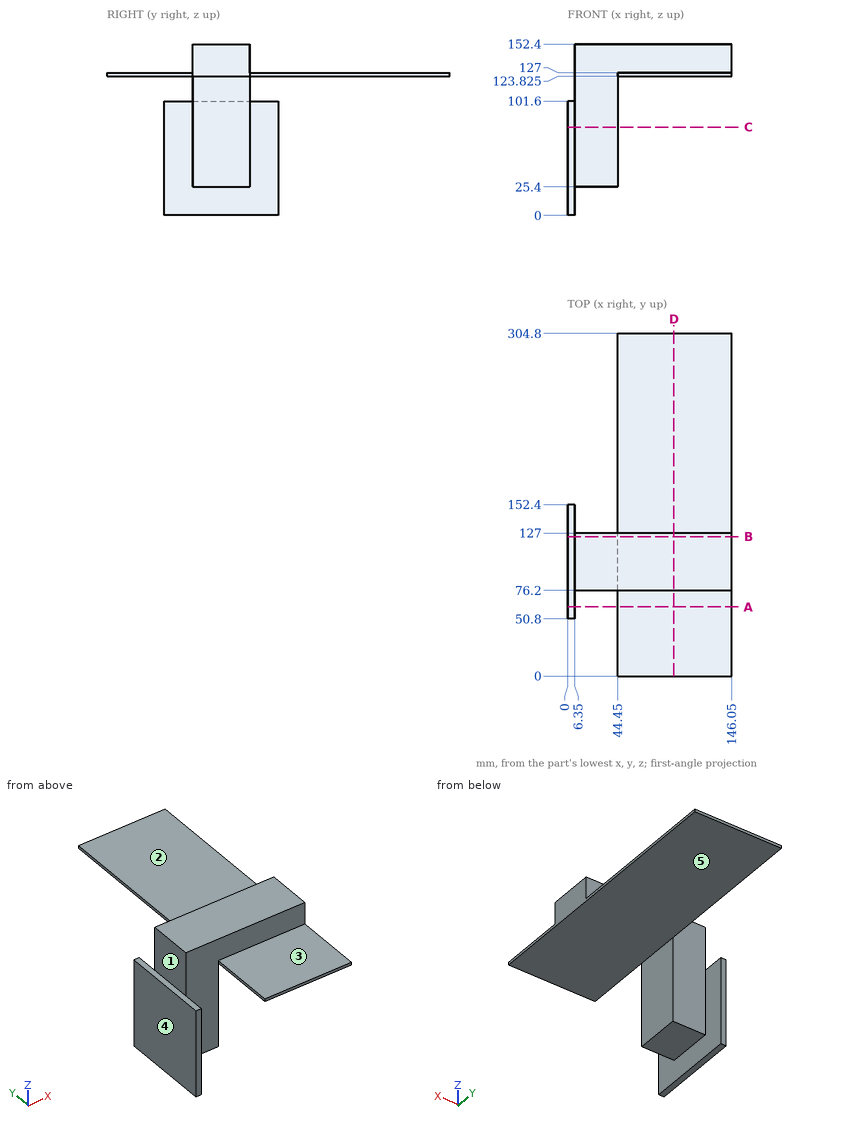
Here's the drawing with two shaded views (mm, measured from the low corner). I have some questions. A direction names the side the tool comes from. Round coordinates to 2 decimals unless told otherwise and drop trailing zeros. Loops run counter-clockwise (first coordinate to the right, second up) from the corner with the lowest first, then second, coordinate; pieces in that order, holes last. Notation, with made-up numbers: (71, 13) - (113, 13) arc R17 cw to (113, 26) - close; hole circle Ø7 at (75.25, -14). An arc over 180 degrees is marked (long way). Use CSV: the item, a comma, the result in double quotes.
Item 1: If we section it at D-D on x = 94.5: List the corners of the cut face in (y, z) for me (3 decimals), then the cut area to 3 significant figures.
Here are the results:
outline,"(0, 123.825) - (304.8, 123.825) - (304.8, 127) - (127, 127) - (127, 152.4) - (76.2, 152.4) - (76.2, 127) - (0, 127) - close"
area,"2,260 mm²"
Item 2: Will these pins go through, and if not, where does the flat tip stop? pin 1 (5 mm diameter, centred on x = 3, y = 86.5, fed in from +Z); pin 2 (19 mm diameter, centred on x = 21.5, y = 99, fed in from -Z); pin 3 (1.5 mm diameter, centred on y = 142, z = 129, fed in from -X); pin 4 (3 mm diameter, centred on y = 129.5, z = 29.5, fed in from +X).
Here are the results:
pin 1,"stops at z = 101.6"
pin 2,"stops at z = 25.4"
pin 3,"passes through"
pin 4,"stops at x = 6.35"
Item 3: If we section it at C-C on z = 78.5: List the corners of the cut face in (x, y) for me.
Here are the results:
outline,"(0, 50.8) - (6.35, 50.8) - (6.35, 76.2) - (44.45, 76.2) - (44.45, 127) - (6.35, 127) - (6.35, 152.4) - (0, 152.4) - close"
Item 4: If we section it at A-A on y = 61.5: List the corners of the cut face in (x, z) for me (3 decimals), then the cut area to 3 significant figures.
Here are the results:
outline,"(0, 0) - (6.35, 0) - (6.35, 101.6) - (0, 101.6) - close; (44.45, 123.825) - (146.05, 123.825) - (146.05, 127) - (44.45, 127) - close"
area,"968 mm²"
Item 5: I need wall thicknesses on L1, parallel to Y at x = 54, z = 142; L2, parallel to X at y = 96.5, z = 14.5; L3, parallel to Z at x = 113, y = 107.5 (3 decimals). Which ranges of each line are inside material? Lowest first, please. Write a range as [from, to].
Here are the results:
L1,"y = [76.2, 127]"
L2,"x = [0, 6.35]"
L3,"z = [123.825, 152.4]"
Item 6: For the marked faces 1, 2, 3, 4 and 5, which set-ups out of +Z, -Z, +X, -X, +Y, -Y let a thin tool reach every point of the face, with its end or its side?
Here are the results:
face 1,"+Z, -X, +Y, -Y"
face 2,"+Z, +X, -X, +Y"
face 3,"+Z, +X, -X, -Y"
face 4,"+Z, -Z, -X, +Y, -Y"
face 5,"-Z, +X, +Y, -Y"
Item 7: If we section it at B-B on y = 124: List the corners of the cut face in (x, z) for me (3 decimals), then the cut area to 3 significant figures.
Here are the results:
outline,"(0, 0) - (6.35, 0) - (6.35, 25.4) - (44.45, 25.4) - (44.45, 123.825) - (146.05, 123.825) - (146.05, 152.4) - (6.35, 152.4) - (6.35, 101.6) - (0, 101.6) - close"
area,"8,390 mm²"
